```python
from build123d import *

# Parameters (mm, degrees)
SKETCH1_R           = 2.2
BOSS_EXTRUDE1_DEPTH = 6.35
FILLET3_R           = 19.05
FILLET4_R           = 6.35
FILLET5_R           = 6.35
FILLET10_R          = 12.7
SKETCH3_R           = 2.2
BOSS_EXTRUDE3_DEPTH = 6.35
FILLET6_R           = 12.7
FILLET8_R           = 3.175
FILLET9_R           = 0.5


with BuildPart() as part:
    # Sketch1 → Boss-Extrude1 (new body)
    with BuildSketch(Plane(origin=(0, 0, 0), x_dir=(1, 0, 0), z_dir=(0, 1, 0))):
        Polygon((63.5, -25.4), (12.7, -25.4), (12.7, 0), (0, 0), (0, -50.8), (63.5, -50.8), align=None)
        with Locations(Location((6.35, -6.35, 0), (0, 0, 270))):
            Circle(SKETCH1_R, mode=Mode.SUBTRACT)
        with Locations(Location((31.75, -31.75, 0), (0, 0, 270))):
            Circle(SKETCH1_R, mode=Mode.SUBTRACT)
        with Locations(Location((57.15, -44.45, 0), (0, 0, 270))):
            Circle(SKETCH1_R, mode=Mode.SUBTRACT)
        with Locations(Location((19.05, -44.45, 0), (0, 0, 270))):
            Circle(SKETCH1_R, mode=Mode.SUBTRACT)
    extrude(amount=BOSS_EXTRUDE1_DEPTH)

    # Fillet3
    fillet3_edges = [part.edges().sort_by_distance(p)[0] for p in [
        (12.7, 3.175, 25.4),
    ]]
    fillet(fillet3_edges, radius=FILLET3_R)

    # Fillet4
    fillet4_edges = [part.edges().sort_by_distance(p)[0] for p in [
        (0, 3.175, 0),
        (12.7, 3.175, 0),
    ]]
    fillet(fillet4_edges, radius=FILLET4_R - 0.0001)  # a hair under: the kernel refuses the full size

    # Fillet5
    fillet5_edges = [part.edges().sort_by_distance(p)[0] for p in [
        (63.5, 3.175, 25.4),
        (63.5, 3.175, 50.8),
    ]]
    fillet(fillet5_edges, radius=FILLET5_R)

    # Fillet10
    fillet10_edges = [part.edges().sort_by_distance(p)[0] for p in [
        (0, 3.175, 50.8),
    ]]
    fillet(fillet10_edges, radius=FILLET10_R)

    # Sketch3 → Boss-Extrude3 (add)
    with BuildSketch(Plane.XZ):
        with BuildLine():
            Line((0, 25.4), (31.75, 25.4))
            Line((31.75, 25.4), (57.15, 25.4))
            ThreePointArc((57.15, 25.4), (61.640128061, 27.259871939), (63.5, 31.75))
            Line((63.5, 31.75), (63.5, 44.45))
            ThreePointArc((63.5, 44.45), (61.640128061, 48.940128061), (57.15, 50.8))
            Line((57.15, 50.8), (12.7, 50.8))
            ThreePointArc((12.7, 50.8), (3.719743879, 47.080256121), (0, 38.1))
            Line((0, 38.1), (0, 25.4))
        make_face()
        with Locations(Location((19.05, 44.45, 0), (0, 0, 270))):
            Circle(SKETCH3_R, mode=Mode.SUBTRACT)
        with Locations(Location((31.75, 31.75, 0), (0, 0, 270))):
            Circle(SKETCH3_R, mode=Mode.SUBTRACT)
        with Locations(Location((57.15, 44.45, 0), (0, 0, 270))):
            Circle(SKETCH3_R, mode=Mode.SUBTRACT)
    extrude(amount=BOSS_EXTRUDE3_DEPTH)

    # Fillet6
    fillet6_edges = [part.edges().sort_by_distance(p)[0] for p in [
        (0, -3.175, 25.4),
    ]]
    fillet(fillet6_edges, radius=FILLET6_R - 0.0001)  # a hair under: the kernel refuses the full size

    # Fillet8
    fillet8_edges = [part.edges().sort_by_distance(p)[0] for p in [
        (22.22495, 0, 25.4),
    ]]
    fillet(fillet8_edges, radius=FILLET8_R)

    # Fillet9
    fillet9_edges = [part.edges().sort_by_distance(p)[0] for p in [
        (3.71971459, -6.35, 29.11971459),
        (18.279615818, 6.35, 19.820384182),
        (0, 0, 17.462416667),
        (1.85984265, 0, 1.85984265),
        (10.84015735, 0, 1.85984265),
        (0, 6.35, 22.22495),
        (1.85984265, 6.35, 1.85984265),
        (10.84015735, 6.35, 1.85984265),
        (63.5, 6.35, 38.1),
        (44.45, 6.35, 25.4),
        (61.640128061, 6.35, 27.259871939),
        (61.640128061, 6.35, 48.940128061),
        (34.925, 6.35, 50.8),
        (3.719743879, 6.35, 47.080256121),
        (34.92495, -6.35, 25.4),
        (61.640128061, -6.35, 27.259871939),
        (63.5, -6.35, 38.1),
        (61.640128061, -6.35, 48.940128061),
        (34.925, -6.35, 50.8),
        (3.719743879, -6.35, 47.080256121),
    ]]
    fillet(fillet9_edges, radius=FILLET9_R)


solid = part.part
```
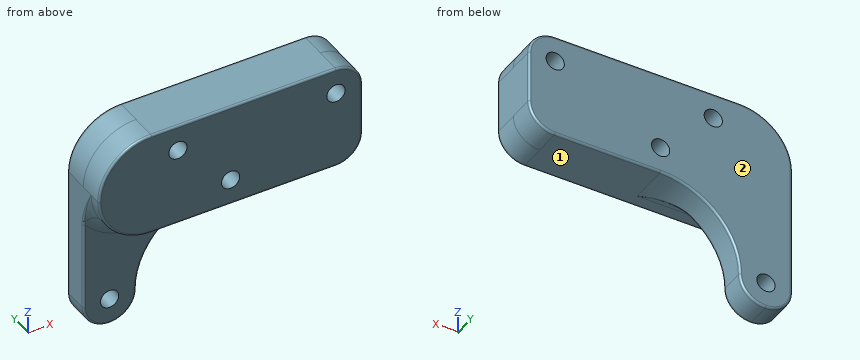
CAD build for the part. Positions are in the model's coordinates, mm. Face numbers are marked on the shaded views. A direction names the side the tool comes from. Coordinates: 2 decimals unless noted, no trailing zeros. Order: outer loops, then holes, each group sorted by start corner. A loop starts at its lowest first (then second) coordinate and runs counter-clockwise, first axis right, second up. Notation, with made-up numbers: M 40,-5 L 75,-5 A17 cw 75,6 Z; hole C -13.75,72.25 d3. An arc over 180 degrees is marked long. Write each question's results on one line, items separated by ' | '. Start each with the question number.
Q1. Drill centre lines: probe 1 along Z at (x, y) = (31.75, 3); probe 2 along Z at (x, y) = (19.05, -5); probe 3 along X at (y, z) = (-2, 44). Where is each one in solid material? Low to high. Write a range as from..to.
Q2. Cut at A-A (y = -4.25). Count the separate pieces of the cut face and the enclosed holes in it, then the cut area to 3 significant figures.
Q3. Cut at B-B (x = 32.5). List the corners of the cut face in (y, z).
Q4. Cut at C-C (x = 44). List the corners of the cut face in (y, z).
Q5. Which spindle directions (+Z, -Z, +X, -X, +Y, -Y) get a long thin tool onto all of the face, cutting with end or side? Do the marked faces 1 and 2. Say none if no direction does.
Q6. Flat gauge pins, fed straight in: P1, Ø3.5, axis at x = 38.5, y = -2.5, coming from the -Z side; P2, Ø1, axis at y = -3.5, z = 43, coming from the -X side; P3, Ø6, axis at x = 14, z = 15, coming from the -Y side. Where does each tip first touch, or does it go through?
Found:
1) probe 1: 25.4..29.55, 33.95..50.8 | probe 2: 25.4..42.25, 46.65..50.8 | probe 3: 1.45..16.9, 21.2..55, 59.3..63.5
2) separate pieces: 1 | enclosed holes: 3 | area: 1,480 mm²
3) outline: M -6.35,25.9 A0.5 ccw -5.85,25.4 L 5.85,25.4 A0.5 ccw 6.35,25.9 L 6.35,29.68 L -6.35,29.68 Z; M -6.35,33.82 L 6.35,33.82 L 6.35,50.3 A0.5 ccw 5.85,50.8 L -5.85,50.8 A0.5 ccw -6.35,50.3 Z
4) outline: M -6.35,25.9 A0.5 ccw -5.85,25.4 L 5.85,25.4 A0.5 ccw 6.35,25.9 L 6.35,50.3 A0.5 ccw 5.85,50.8 L -5.85,50.8 A0.5 ccw -6.35,50.3 Z
5) face 1: -Z, +X, -Y | face 2: +Z, -Z, +X, -X, +Y
6) P1: z = 25.4 | P2: x = 0.79 | P3: y = 0
